For this review, take the finished solid that the model builds, in its own axes (mm). Give positions to 0.01 mm unless a question says otherwise; leave off trailing zeros. Write each loop counter-clockwise with the first axis right and the second up, starting at its lowest first coordinate (ties: lowest second). Pieces come first, ordered by that corner, then holes. Notation, with made-up numbers: M 73,89.25 L 78,89.25 A17 ccw 78,95.25 Z; hole C 56.5,-2 d2. An arc over 180 degrees is marked long. Use one line per item in the form item = value. Start each with the question number.
Q1. Consider section C-C on x = -1. Write out the cut boundary in (y, z).
Q2. Consider section A-A on x = 5.08. Write out the cut boundary in (y, z), and give its area (3 significant figures).
Q3. Consider section B-B on y = 14.5. Write out the cut boundary in (x, z).
Q4. For probe 1 along Y at (x, z) = (5.08, 1.55); probe 2 along X at (y, z) = (8, 1.6); probe 3 along X at (y, z) = (-20, 1.4), list the stretches that pass through material, from the lowest coordinate up. Write a range as [from, to].
Q5. Clearance check with flat-ended pins moving along their axes: pin 1 Ø0.9 at (x, z) = (-8, 1.5) entering from +Y; pin 2 Ø0.9 at (y, z) = (3.5, 1.5) entering from -X; pin 3 Ø1.5 at (y, z) = (-22.5, 2) entering from +X. State where each tip first meets the part, or that it passes through.
Q6. Consider section D-D on z = 1.05. Give the number of separate pieces and of enclosed holes in the cut face, and give its area (3 significant figures).
```python
from build123d import *

# Parameters (mm, degrees)
F0_W      = 50.8
F0_H      = 88.9
F1_DEPTH  = 2.9718
F2_W      = 20.32
F2_H      = 41.402
F3_DEPTH  = 25.4
F4_W      = 12.7
F4_H      = 2.9718
F5_DEPTH  = 25.4
F6_W      = 2.9718
F6_H      = 6.35
F7_DEPTH  = 25.4
F8_R      = 1.8415
F9_DEPTH  = 25.4
F11_DEPTH = 25.4
F12_R     = 19.05


with BuildPart() as f1:
    # F0 (on Top) → F1 (new body)
    with BuildSketch(Plane.XY):
        Rectangle(F0_W, F0_H)
    extrude(amount=F1_DEPTH)

    # F2 (on face) → F3 (cut)
    with BuildSketch(Plane.XY.offset(2.9718)):
        with Locations((0, 13.589)):
            Rectangle(F2_W, F2_H)
    extrude(amount=-F3_DEPTH, mode=Mode.SUBTRACT)

    # F4 (on face) → F5 (cut)
    with BuildSketch(Plane.XY.offset(2.9718)):
        with Locations((-12.7, -42.9641)):
            Rectangle(F4_W, F4_H)
        with Locations((12.7, -42.9641)):
            Rectangle(F4_W, F4_H)
    extrude(amount=-F5_DEPTH, mode=Mode.SUBTRACT)

    # F6 (on face) → F7 (cut)
    with BuildSketch(Plane.XY.offset(2.9718)):
        with Locations((23.9141, 3.175)):
            Rectangle(F6_W, F6_H)
        with Locations((-23.9141, 3.175)):
            Rectangle(F6_W, F6_H)
        with Locations((-23.9141, -22.225)):
            Rectangle(F6_W, F6_H)
        with Locations((23.9141, -22.225)):
            Rectangle(F6_W, F6_H)
    extrude(amount=-F7_DEPTH, mode=Mode.SUBTRACT)

    # F8 (on face) → F9 (cut)
    with BuildSketch(Plane.XY.offset(2.9718)):
        with Locations((-5.08, 38.354)):
            Circle(F8_R)
        with Locations((5.08, 38.354)):
            Circle(F8_R)
        with Locations((-5.08, -9.906)):
            Circle(F8_R)
        with Locations((5.08, -9.906)):
            Circle(F8_R)
    extrude(amount=-F9_DEPTH, mode=Mode.SUBTRACT)

    # F10 (on face) → F11 (cut)
    with BuildSketch(Plane.XY.offset(2.9718)):
        with BuildLine():
            ThreePointArc((2.8575, 34.29), (0, 37.1475), (-2.8575, 34.29))
            Line((-2.8575, 34.29), (2.8575, 34.29))
        make_face()
        with BuildLine():
            ThreePointArc((-2.8575, -7.112), (0, -9.9695), (2.8575, -7.112))
            Line((2.8575, -7.112), (-2.8575, -7.112))
        make_face()
    extrude(amount=-F11_DEPTH, mode=Mode.SUBTRACT)

    # F12
    f12_edges = [f1.edges().sort_by_distance(p)[0] for p in [
        (25.4, 44.45, 1.4859),
        (-25.4, 44.45, 1.4859),
    ]]
    fillet(f12_edges, radius=F12_R)


solid = f1.part
```
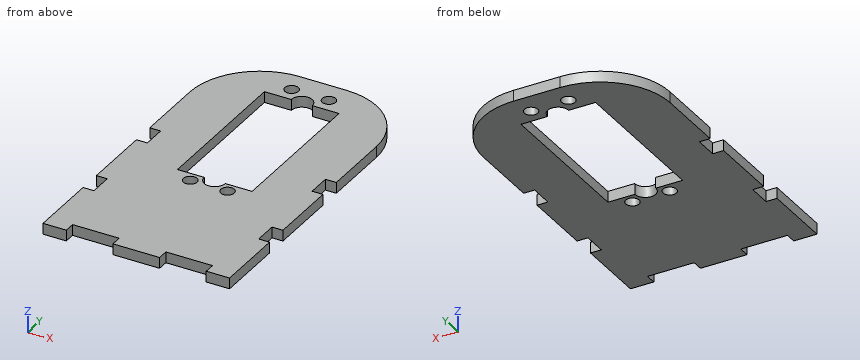
Working result:
q1.outline = M -44.45,0 L -9.79,0 L -9.79,2.97 L -44.45,2.97 Z; M 36.97,0 L 44.45,0 L 44.45,2.97 L 36.97,2.97 Z
q2.outline = M -44.45,0 L -11.75,0 L -11.75,2.97 L -44.45,2.97 Z; M -8.06,0 L -7.11,0 L -7.11,2.97 L -8.06,2.97 Z; M 34.29,0 L 36.51,0 L 36.51,2.97 L 34.29,2.97 Z; M 40.2,0 L 44.45,0 L 44.45,2.97 L 40.2,2.97 Z
q2.area = 119 mm²
q3.outline = M -25.4,0 L -10.16,0 L -10.16,2.97 L -25.4,2.97 Z; M 10.16,0 L 25.4,0 L 25.4,2.97 L 10.16,2.97 Z
q4.probe_1 = [-44.45, -11.75], [-8.06, -7.11], [34.29, 36.51], [40.2, 44.45]
q4.probe_2 = [-25.4, -10.16], [10.16, 25.4]
q4.probe_3 = [-22.43, 22.43]
q5.pin_1 = 44.41
q5.pin_2 = -22.43
q5.pin_3 = 22.43
q6.separate_pieces = 1
q6.enclosed_holes = 5
q6.area = 3,300 mm²
